Geometry: see drawing. Coordinates: mm, zero at the bounding-box minimum. Give positions to 0.01 mm unless a question says otherwise; leave off trailing zeros. Order: outer loops, then holes, each group sorted by start corner. A loop starts at its lowest first (then second) coordinate and runs counter-clockwise, first axis right, second up. Notation, with made-up numbers: M -14.75,-37 L 1.25,-37 A25 ccw 1.25,1 Z; hole C -13,27 d8. An arc over 180 degrees is marked long. Use a Markdown table: item, result.
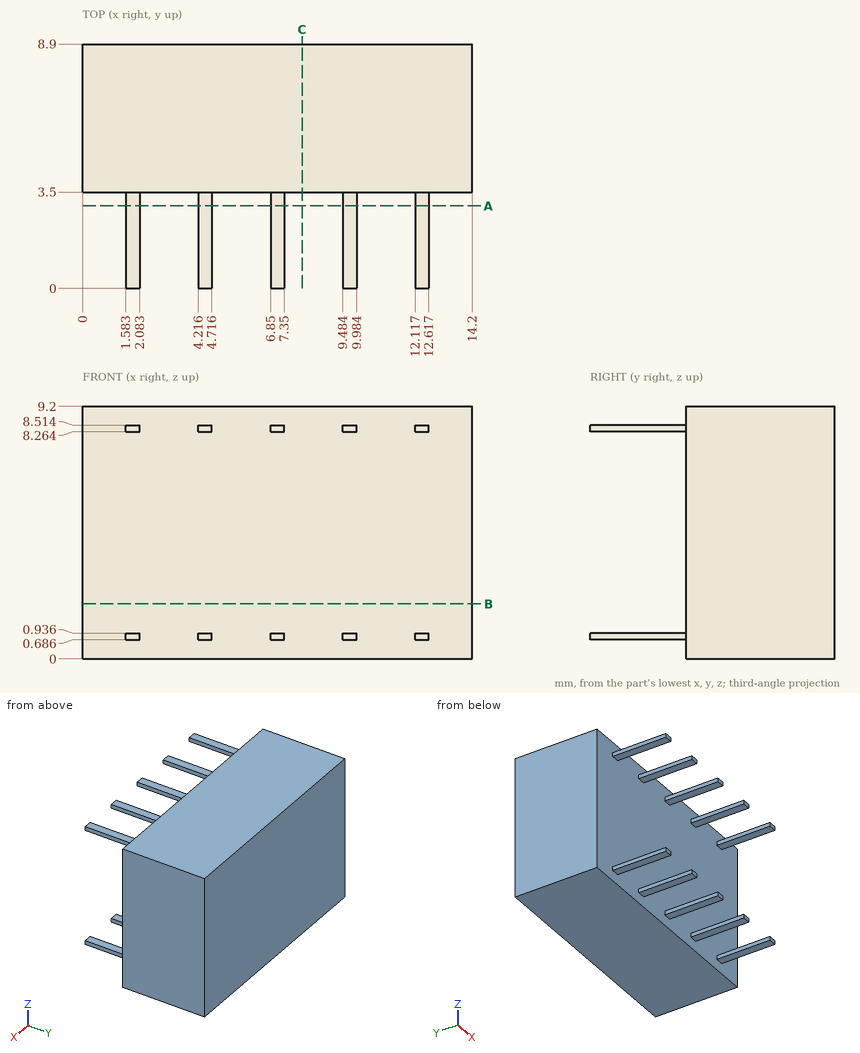
1) Cut plane C-C on x = 8. Return loops of the section in (y, z), and give its area (3 significant figures).
Response values:
| item | result |
|---|---|
| outline | M 3.5,0 L 8.9,0 L 8.9,9.2 L 3.5,9.2 Z |
| area | 49.7 mm² |
2) Cut plane A-A on y = 3. State how many separate pieces and enclosed holes the cut face has.
Response values:
| item | result |
|---|---|
| separate pieces | 10 |
| enclosed holes | 0 |
3) Material intervals for line 1 (Z direction, x = 7.25, y = 1) (1 decimal); line 2 (Y direction, x = 3, z = 8.75), sorted ascending. Write a range as from..to.
Response values:
| item | result |
|---|---|
| line 1 | z = 0.7..0.9, 8.3..8.5 |
| line 2 | y = 3.5..8.9 |
4) Cut plane B-B on z = 2. Return loops of the section in (x, y).
Response values:
| item | result |
|---|---|
| outline | M 0,3.5 L 14.2,3.5 L 14.2,8.9 L 0,8.9 Z |
